Check sheet for the modelled part. Datum: model origin and axes. Units: mm. Give positions to 0.01 mm unless a question says otherwise; leave off trailing zeros. Loops run counter-clockwise (first coordinate to the right, second up) from the corner with the lowest first, then second, coordinate; pieces in that order, holes last. Notation, with made-up numbers: M 83,-18 L 136,-18 A9 ccw 136,-12 Z; hole C 11,9.5 d6. An arc over 180 degrees is marked long. Put each result on its own line as item: value. Start each with the question number.
```python
from build123d import *

# Parameters (mm, degrees)
BOSS_EXTRUDE1_DEPTH = 8
BOSS_EXTRUDE2_DEPTH = 0.6
CUT_EXTRUDE1_DEPTH  = 0.6
SKETCH4_R           = 1.1
CUT_EXTRUDE2_DEPTH  = 13.5
CUT_EXTRUDE3_START  = -13.5
SKETCH5_R           = 1.1
CUT_EXTRUDE3_DEPTH  = 13.5
CUT_EXTRUDE6_START  = -3.6
CUT_EXTRUDE6_DEPTH  = 1.8
CUT_EXTRUDE7_START  = -3.6
CUT_EXTRUDE7_DEPTH  = 1.8
SKETCH8_W           = 295.2
SKETCH8_H           = 19.1
CUT_EXTRUDE8_DEPTH  = 1.2
SKETCH9_W           = 24.86
SKETCH9_H           = 10
CUT_EXTRUDE9_DEPTH  = 1.6
BOSS_EXTRUDE3_DEPTH = 238.72
SKETCH11_R          = 1.1
CUT_EXTRUDE10_DEPTH = 1.2
CUT_EXTRUDE11_REACH = 151.204
SKETCH12_R          = 2
CHAMFER1_SIZE       = 0.9


with BuildPart() as part:
    # Sketch1 → Boss-Extrude1 (new body)
    with BuildSketch(Plane(origin=(0, 0, 0), x_dir=(1, 0, 0), z_dir=(0, 1, 0))):
        with BuildLine():
            Line((-118.36, 0), (120.36, 0))
            Line((120.36, 0), (120.36, 1.3))
            Line((120.36, 1.3), (145.3, 1.3))
            ThreePointArc((145.3, 1.3), (146.488640518, 1.452788358), (147.6, 1.901219694))
            Line((147.6, 1.901219694), (147.6, 11.6))
            Line((147.6, 11.6), (134.1, 11.6))
            Line((134.1, 11.6), (134.1, 11.2))
            Line((134.1, 11.2), (95.6, 11.2))
            Line((95.6, 11.2), (95.6, 1.2))
            Line((95.6, 1.2), (-93.6, 1.2))
            Line((-93.6, 1.2), (-93.6, 11.2))
            Line((-93.6, 11.2), (-134.1, 11.2))
            Line((-134.1, 11.2), (-134.1, 11.6))
            Line((-134.1, 11.6), (-147.6, 11.6))
            Line((-147.6, 11.6), (-147.6, 1.901219694))
            ThreePointArc((-147.6, 1.901219694), (-146.488640518, 1.452788358), (-145.3, 1.3))
            Line((-145.3, 1.3), (-118.36, 1.3))
            Line((-118.36, 1.3), (-118.36, 0))
        make_face()
    extrude(amount=BOSS_EXTRUDE1_DEPTH)

    # Sketch2 → Boss-Extrude2 (add)
    with BuildSketch(Plane.XZ):
        Polygon((120.36, -1.2), (120.36, -11.341421356), (129.318578644, -20.3), (-127.318578644, -20.3), (-118.36, -11.341421356), (-118.36, -1.2), align=None)
    extrude(amount=-BOSS_EXTRUDE2_DEPTH)

    # Sketch3 → Cut-Extrude1 (cut)
    with BuildSketch(Plane.XZ):
        Polygon((-118.36, -11.2), (-134.1, -11.2), (-134.1, -11.6), (-147.6, -11.6), (-147.6, -1.3), (-118.36, -1.3), align=None)
        Polygon((120.36, -1.3), (147.6, -1.3), (147.6, -11.6), (134.1, -11.6), (134.1, -11.2), (120.36, -11.2), align=None)
    extrude(amount=-CUT_EXTRUDE1_DEPTH, mode=Mode.SUBTRACT)

    # Sketch4 → Cut-Extrude2 (cut)
    with BuildSketch(Plane(origin=(147.6, 0, 0), x_dir=(0, 0, -1), z_dir=(1, 0, 0))):
        with Locations((8, 4)):
            Circle(SKETCH4_R)
    extrude(amount=-CUT_EXTRUDE2_DEPTH, mode=Mode.SUBTRACT)

    # Sketch5 → Cut-Extrude3 (cut)
    with BuildSketch(Plane.ZY.offset(147.6).offset(CUT_EXTRUDE3_START)):
        with Locations(Location((-8, 4, 0), (0, 0, 180))):
            Circle(SKETCH5_R)
    extrude(amount=CUT_EXTRUDE3_DEPTH, mode=Mode.SUBTRACT)

    # Sketch6 → Cut-Extrude6 (cut)
    with BuildSketch(Plane(origin=(147.6, 0, 0), x_dir=(0, 0, -1), z_dir=(1, 0, 0)).offset(CUT_EXTRUDE6_START)):
        Polygon((5.6, 5.385640646), (5.6, 2.614359354), (8, 1.228718708), (10.4, 2.614359354), (10.4, 5.385640646), (10.4, 8), (5.6, 8), align=None)
    extrude(amount=-CUT_EXTRUDE6_DEPTH, mode=Mode.SUBTRACT)

    # Sketch7 → Cut-Extrude7 (cut)
    with BuildSketch(Plane.ZY.offset(147.6).offset(CUT_EXTRUDE7_START)):
        Polygon((-10.4, 8), (-10.4, 2.614359354), (-8, 1.228718708), (-5.6, 2.614359354), (-5.6, 8), align=None)
    extrude(amount=-CUT_EXTRUDE7_DEPTH, mode=Mode.SUBTRACT)

    # Sketch8 → Cut-Extrude8 (cut)
    with BuildSketch(Plane(origin=(0, 8, 0), x_dir=(1, 0, 0), z_dir=(0, 1, 0))):
        with Locations((0, 10.75)):
            Rectangle(SKETCH8_W, SKETCH8_H)
    extrude(amount=-CUT_EXTRUDE8_DEPTH, mode=Mode.SUBTRACT)

    # Sketch9 → Cut-Extrude9 (cut)
    with BuildSketch(Plane(origin=(0, 6.8, 0), x_dir=(1, 0, 0), z_dir=(0, 1, 0))):
        with Locations((108.03, 6.2)):
            Rectangle(SKETCH9_W, SKETCH9_H)
        with Locations((-106.03, 6.2)):
            Rectangle(SKETCH9_W, SKETCH9_H)
    extrude(amount=-CUT_EXTRUDE9_DEPTH, mode=Mode.SUBTRACT)

    # Sketch10 → Boss-Extrude3 (add)
    with BuildSketch(Plane.ZY.offset(118.36)):
        with BuildLine():
            Line((0, 8), (2.113102916, 3.253893145))
            ThreePointArc((2.113102916, 3.253893145), (1.939911372, 1.053285936), (0, 0))
            Line((0, 0), (0, 8))
        make_face()
    extrude(amount=-BOSS_EXTRUDE3_DEPTH)

    # Sketch11 → Cut-Extrude10 (cut)
    with BuildSketch(Plane(origin=(0, 0, -1.2), x_dir=(-1, 0, 0), z_dir=(0, 0, -1))):
        with Locations((73.7, 5.8)):
            Circle(SKETCH11_R)
        with Locations((-73.7, 5.8)):
            Circle(SKETCH11_R)
        with Locations((60, 5.8)):
            Circle(SKETCH11_R)
        with Locations((0, 5.8)):
            Circle(SKETCH11_R)
        with Locations((-60, 5.8)):
            Circle(SKETCH11_R)
    extrude(amount=-CUT_EXTRUDE10_DEPTH, mode=Mode.SUBTRACT)

    # Sketch12 → Cut-Extrude11 (cut, up to next)
    with BuildSketch(Plane(origin=(0, 0, 0), x_dir=(-1, 0, 0), z_dir=(0, 0, -1)), mode=Mode.PRIVATE) as cut_extrude11_sk1:
        with Locations((-73.7, 5.8)):
            Circle(SKETCH12_R)
    cut_extrude11_tool1 = extrude(cut_extrude11_sk1.sketch, amount=-CUT_EXTRUDE11_REACH, mode=Mode.PRIVATE) & part.part
    # Sketch12 → Cut-Extrude11 (cut, up to next)
    with BuildSketch(Plane(origin=(0, 0, 0), x_dir=(-1, 0, 0), z_dir=(0, 0, -1)), mode=Mode.PRIVATE) as cut_extrude11_sk2:
        with Locations((73.7, 5.8)):
            Circle(SKETCH12_R)
    cut_extrude11_tool2 = extrude(cut_extrude11_sk2.sketch, amount=-CUT_EXTRUDE11_REACH, mode=Mode.PRIVATE) & part.part
    # Sketch12 → Cut-Extrude11 (cut, up to next)
    with BuildSketch(Plane(origin=(0, 0, 0), x_dir=(-1, 0, 0), z_dir=(0, 0, -1)), mode=Mode.PRIVATE) as cut_extrude11_sk3:
        with Locations((-60, 5.8)):
            Circle(SKETCH12_R)
    cut_extrude11_tool3 = extrude(cut_extrude11_sk3.sketch, amount=-CUT_EXTRUDE11_REACH, mode=Mode.PRIVATE) & part.part
    # Sketch12 → Cut-Extrude11 (cut, up to next)
    with BuildSketch(Plane(origin=(0, 0, 0), x_dir=(-1, 0, 0), z_dir=(0, 0, -1)), mode=Mode.PRIVATE) as cut_extrude11_sk4:
        with Locations((0, 5.8)):
            Circle(SKETCH12_R)
    cut_extrude11_tool4 = extrude(cut_extrude11_sk4.sketch, amount=-CUT_EXTRUDE11_REACH, mode=Mode.PRIVATE) & part.part
    # Sketch12 → Cut-Extrude11 (cut, up to next)
    with BuildSketch(Plane(origin=(0, 0, 0), x_dir=(-1, 0, 0), z_dir=(0, 0, -1)), mode=Mode.PRIVATE) as cut_extrude11_sk5:
        with Locations((60, 5.8)):
            Circle(SKETCH12_R)
    cut_extrude11_tool5 = extrude(cut_extrude11_sk5.sketch, amount=-CUT_EXTRUDE11_REACH, mode=Mode.PRIVATE) & part.part
    add(cut_extrude11_tool1.solids().sort_by_distance((73.7, 5.8, 0))[0], mode=Mode.SUBTRACT)
    add(cut_extrude11_tool2.solids().sort_by_distance((-73.7, 5.8, 0))[0], mode=Mode.SUBTRACT)
    add(cut_extrude11_tool3.solids().sort_by_distance((60, 5.8, 0))[0], mode=Mode.SUBTRACT)
    add(cut_extrude11_tool4.solids().sort_by_distance((0, 5.8, 0))[0], mode=Mode.SUBTRACT)
    add(cut_extrude11_tool5.solids().sort_by_distance((-60, 5.8, 0))[0], mode=Mode.SUBTRACT)

    # Chamfer1
    chamfer1_edges = [part.edges().sort_by_distance(p)[0] for p in [
        (74.8, 5.8, 0),
        (-58.9, 5.8, 0),
        (1.1, 5.8, 0),
        (61.1, 5.8, 0),
        (-72.6, 5.8, 0),
    ]]
    chamfer(chamfer1_edges, length=CHAMFER1_SIZE - 0.0001)  # a hair under: the kernel refuses the full size


solid = part.part
```
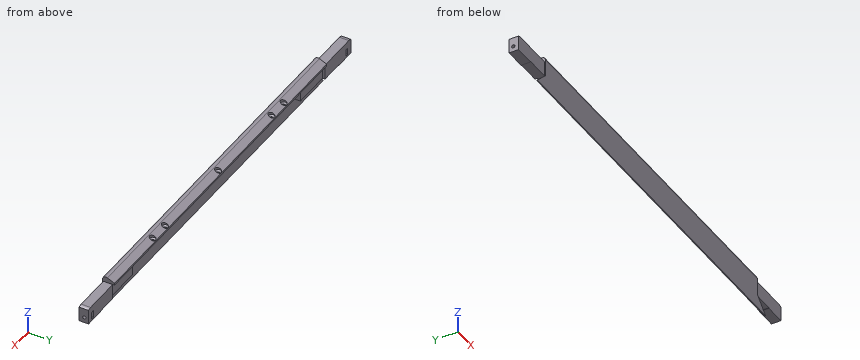
Q1. Section check A-A, the plane x = 11. Record the cut outline in (y, z), then the cut area to 3 significant figures.
Q2. Depth check by flat-ended pin: P1, Ø1.4, axis at y = 4.5, z = -8, coming from the +X side; P2, Ø1.5, axis at x = -57, y = 3.5, coming from the -Z side; P3, Ø1, axis at x = -45, z = -5, coming from the +Y side; P4, Ø0.5, axis at x = 143.5, y = 5, coming from the -Z side. Enter the tip coordinate at first touch or a pass-through.
Q3. Section check B-B, the plane z = -14. Record the cut outline in (x, y).
Q4. Thickness scan on line 1 along X through (y, z) = (1.75, -6); line 2 along Y through (x, z) = (-73.7, -1); line 3 along X through (y, z) = (6.25, -1). Record the ranges inside material, lowest first. Write a range as [from, to].
Found:
1. outline: M 0,-20.3 L 0.6,-20.3 L 0.6,-1.2 L 8,-1.2 L 8,0 L 3.25,2.11 A2.31 ccw 0,0 Z
1. area: 32.4 mm^2
2. P1: stops at x = 147.6
2. P2: stops at z = -1.2
2. P3: stops at y = 0.6
2. P4: stops at z = -11.6
3. outline: M -121.02,0 L 123.02,0 L 123.02,0.6 L -121.02,0.6 Z
4. line 1: x = [-147.6, -93.6], [95.6, 147.6]
4. line 2: y = [0, 4.7], [6.9, 8]
4. line 3: x = [-118.36, -74.7], [-72.7, -61], [-59, -1], [1, 59], [61, 72.7], [74.7, 120.36]
